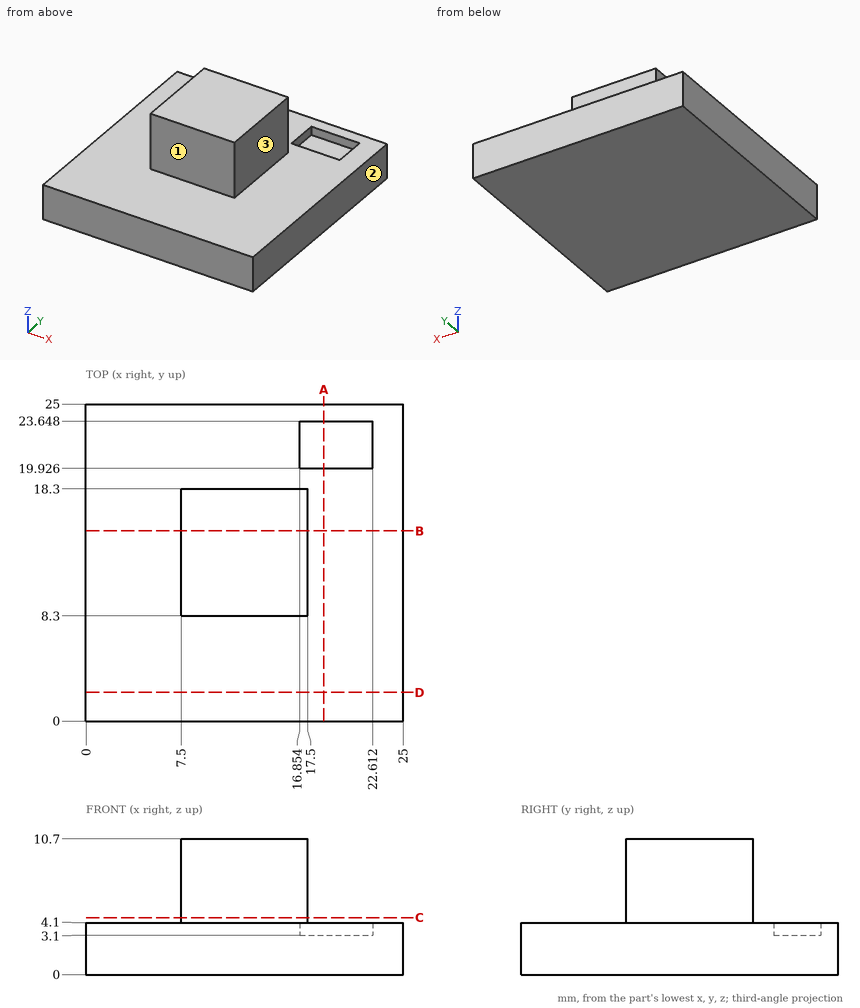
Source: three-view drawing plus pictorial views. Frame: mm from the lowest corner of the part. A direction names the side the tool comes from. Give positions to 0.01 mm unless a question says otherwise; leave off trailing zeros. Loops run counter-clockwise (first coordinate to the right, second up) from the corner with the lowest first, then second, coordinate; pieces in that order, holes last.
1) Section query A-A on x = 18.75. Return the cut outline in (y, z).
A:
outline: (0, 0) - (25, 0) - (25, 4.1) - (23.65, 4.1) - (23.65, 3.1) - (19.93, 3.1) - (19.93, 4.1) - (0, 4.1) - close
2) Section query D-D on y = 2.25. Return the cut outline in (x, z), and give its area (4 significant figures).
A:
outline: (0, 0) - (25, 0) - (25, 4.1) - (0, 4.1) - close
area: 102.5 mm2
3) Contact query for flat-ended pins moving along their axis: pin 1 (5 mm diameter, centred on y = 6, z = 7.5, fed in from -X); pin 2 (6 mm diameter, centred on y = 22.5, z = 9.5, fed in from -X); pin 3 (2 mm diameter, centred on x = 12, z = 6, fed in from -Y); pin 4 (1.9 mm diameter, centred on x = 20, y = 22, fed in from +Z). Output: stop coordinate, or through.
A:
pin 1: stops at x = 7.5
pin 2: passes through
pin 3: stops at y = 8.3
pin 4: stops at z = 3.1
4) Section query C-C on z = 4.5. Return the cut outline in (x, y), and give its area (3 significant figures).
A:
outline: (7.5, 8.3) - (17.5, 8.3) - (17.5, 18.3) - (7.5, 18.3) - close
area: 100 mm2
5) Line query: L1, parallel to X at y = 23.5, z = 4; L2, parallel to X at y = 9.75, z = 6.25; L3, parallel to Y at x = 14.25, z = 7.75. Output: solid intervals per line, ascending.
A:
L1: x = 0 to 16.85, 22.61 to 25
L2: x = 7.5 to 17.5
L3: y = 8.3 to 18.3
6) Reachability of the marked faces 1, 2 and 3 from +Z, -Z, +X, -X, +Y, -Y: full face, straight path, thin tool, end or side. Return the list, or none.
A:
face 1: +Z, +X, -X, -Y
face 2: +Z, -Z, +X, +Y, -Y
face 3: +Z, +X, +Y, -Y
7) Section query B-B on y = 15. Return the cut outline in (x, z), and give its area (4 significant figures).
A:
outline: (0, 0) - (25, 0) - (25, 4.1) - (17.5, 4.1) - (17.5, 10.7) - (7.5, 10.7) - (7.5, 4.1) - (0, 4.1) - close
area: 168.5 mm2
